The model under review builds one solid part; all positions refer to its coordinate system, in mm. Coordinates: 2 decimals unless noted, no trailing zeros. Order: outer loops, then holes, each group sorted by start corner. A loop starts at its lowest first (then second) coordinate and runs counter-clockwise, first axis right, second up.
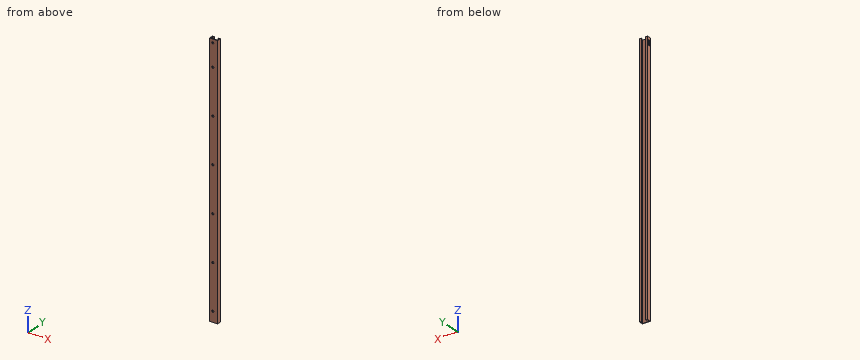
```python
from build123d import *

# Parameters (mm, degrees)
BOSS_EXTRU_1_DEPTH         = 813
D_GAGEMENT_M61_D           = 6.6
R_P_TITION_LIN_AIRE1_COUNT = 12
R_P_TITION_LIN_AIRE1_PITCH = 70
CUT_EXTRUDE1_DEPTH         = 5


with BuildPart() as part:
    # Esquisse1 → Boss.-Extru.1 (new body)
    with BuildSketch(Plane.XY):
        Polygon((-6.5, 12.5), (-12.5, 12.5), (-12.5, 0), (12.5, 0), (12.5, 12.5), (6.5, 12.5), (6.5, 10.5), (10.5, 10.5), (10.5, 2), (-10.5, 2), (-10.5, 10.5), (-6.5, 10.5), align=None)
    extrude(amount=BOSS_EXTRU_1_DEPTH)

    # Dégagement M61 (through all)
    with Locations(Plane(origin=(0, 0, 0), x_dir=(-1, 0, 0), z_dir=(0, -1, 0))):
        with Locations((2.40627347, -801.806864395)):
            d_gagement_m61 = Hole(D_GAGEMENT_M61_D / 2)

    # Répétition linéaire1: Dégagement M61 ×12, 5 skipped
    with Locations(*[(0, 0, -i * R_P_TITION_LIN_AIRE1_PITCH) for i in range(1, R_P_TITION_LIN_AIRE1_COUNT) if i not in (2, 4, 6, 8, 10)]):
        add(d_gagement_m61, mode=Mode.SUBTRACT)

    # Sketch1 → Cut-Extrude1 (cut)
    with BuildSketch(Plane(origin=(-12.5, 0, 0), x_dir=(0, 0, -1), z_dir=(1, 0, 0))):
        with BuildLine():
            Line((-803, 8.949119862), (-789.837109693, 8.949119862))
            ThreePointArc((-789.837109693, 8.949119862), (-787.337109693, 6.449119862), (-789.837109693, 3.949119862))
            Line((-789.837109693, 3.949119862), (-803, 3.949119862))
            ThreePointArc((-803, 3.949119862), (-805.5, 6.449119862), (-803, 8.949119862))
        make_face()
    extrude(amount=CUT_EXTRUDE1_DEPTH, mode=Mode.SUBTRACT)


solid = part.part
```
(1) Wall thickness on probe 1 along X at (y, z) = (4, 463); probe 2 along Y at (x, z) = (-8.25, 315.5); probe 3 along X at (y, z) = (11.25, 594): over which ranges is each line inside the solid? List them lowest first.
A:
probe 1: x = -12.5 to -10.5, 10.5 to 12.5
probe 2: y = 0 to 2, 10.5 to 12.5
probe 3: x = -12.5 to -6.5, 6.5 to 12.5
(2) For pin 1 Ø6 at (x, z) = (-2.41, 801.81) entering from -Y; pin 2 Ø4 at (x, z) = (4, 428) entering from +Y, all flat-tipped, find the tip position at first contact; note any pin that passes through.
A:
pin 1: passes through
pin 2: stops at y = 2
(3) We need section A-A, the plane z = 392. Write out the cut boundary in (x, y).
A:
outline: (-12.5, 0) - (12.5, 0) - (12.5, 12.5) - (6.5, 12.5) - (6.5, 10.5) - (10.5, 10.5) - (10.5, 2) - (-10.5, 2) - (-10.5, 10.5) - (-6.5, 10.5) - (-6.5, 12.5) - (-12.5, 12.5) - close
